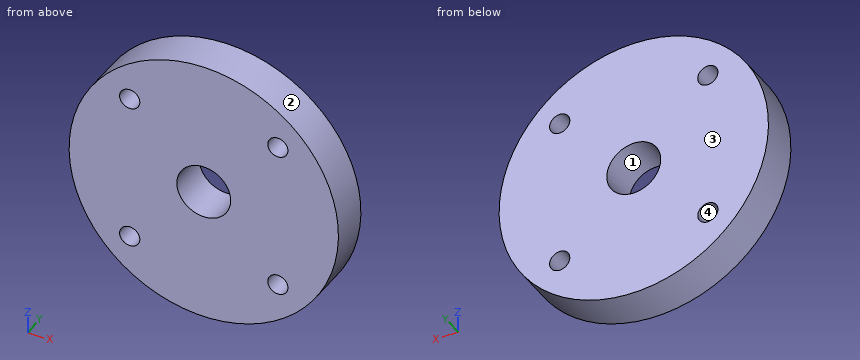
```python
from build123d import *

# Parameters (mm, degrees)
SKETCH1_R                         = 20
ARM_DISTANS_BOSS_EXTRUDE1_DEPTH   = 6
SKETCH2_R                         = 1.5
MOUNTING_HOLES_CUT_EXTRUDE1_DEPTH = 6
SKETCH3_R                         = 4
CUT_EXTRUDE1_DEPTH                = 6


with BuildPart() as part:
    # Sketch1 → Arm Distans Boss-Extrude1 (new body)
    with BuildSketch(Plane(origin=(0, 0, 0), x_dir=(1, 0, 0), z_dir=(0, 1, 0))):
        with Locations(Location((0, 0, 0), (0, 0, 270))):
            Circle(SKETCH1_R)
    extrude(amount=ARM_DISTANS_BOSS_EXTRUDE1_DEPTH)

    # Sketch2 → Mounting Holes Cut-Extrude1 (cut)
    with BuildSketch(Plane(origin=(0, 6, 0), x_dir=(1, 0, 0), z_dir=(0, 1, 0))):
        with Locations(Location((11, 11, 0), (0, 0, 270))):
            Circle(SKETCH2_R)
        with Locations(Location((-11, 11, 0), (0, 0, 270))):
            Circle(SKETCH2_R)
        with Locations(Location((-11, -11, 0), (0, 0, 270))):
            Circle(SKETCH2_R)
        with Locations(Location((11, -11, 0), (0, 0, 270))):
            Circle(SKETCH2_R)
    extrude(amount=-MOUNTING_HOLES_CUT_EXTRUDE1_DEPTH, mode=Mode.SUBTRACT)

    # Sketch3 → Cut-Extrude1 (cut)
    with BuildSketch(Plane.XZ):
        with Locations(Location((0, 0, 0), (0, 0, 270))):
            Circle(SKETCH3_R)
    extrude(amount=-CUT_EXTRUDE1_DEPTH, mode=Mode.SUBTRACT)


solid = part.part
```
Work out the finished part from the listing and answer in its coordinate system (mm). Face numbers are marked on the shaded views. Coordinates: 2 decimals unless noted, no trailing zeros. Loops run counter-clockwise (first coordinate to the right, second up) from the corner with the lowest first, then second, coordinate; pieces in that order, holes last. Notation, with made-up numbers: M -31,-15 L -19,-15 A15 cw -19,4 Z; hole C -1.5,59.5 d7. An arc over 180 degrees is marked long. Use CSV: the item, a comma, the result in double quotes. Start each with the question number.
(1) Consider line 1 (X direction, y = 1.8, z = -11); line 2 (X direction, y = 4.4, z = 0); line 3 (X direction, y = 3.75, z = -10.5). Determine where each line is inside the solid, lowest interval first.
(2) For a pull along Z with two mould halves and no side action, classify the marked faces 1, 2, 3 and 4 as +Z half, -Z half, draft (parallel to the pull), parting line (faces both ways), or undercut.
(3) Find section B-B, the plane z = -3. Give the vertices of the cut face in (x, y), then the cut area to 3 significant figures.
(4) Find section D-D, the plane x = 11. Give the vertices of the cut face in (y, z), then the cut area to 3 significant figures.
(5) Find section C-C, the plane y = 1.6. Give the vertices of the cut face in (x, z).
(6) Given pin 1 Ø3 at (x, y) = (2, 5.5) entering from -Z; pin 2 Ø1 at (x, y) = (12.5, 2) entering from +Z; pin 3 Ø1.5 at (y, z) = (1, 10.5) entering from -X, each flat-ended and moving along its own axis, determine where each tip first touches the part or whether it passes through.
(7) Find section A-A, the plane x = 0. Give the vertices of the cut face in (y, z), then the cut area to 3 significant figures.
Recorded:
1,line 1,"x = -16.7 to -12.5, -9.5 to 9.5, 12.5 to 16.7"
1,line 2,"x = -20 to -4, 4 to 20"
1,line 3,"x = -17.02 to -12.41, -9.59 to 9.59, 12.41 to 17.02"
2,face 1,"undercut"
2,face 2,"parting line"
2,face 3,"draft"
2,face 4,"undercut"
3,outline,"M -19.77,0 L -2.65,0 L -2.65,6 L -19.77,6 Z; M 2.65,0 L 19.77,0 L 19.77,6 L 2.65,6 Z"
3,area,"206 mm^2"
4,outline,"M 0,-16.7 L 6,-16.7 L 6,-12.5 L 0,-12.5 Z; M 0,-9.5 L 6,-9.5 L 6,9.5 L 0,9.5 Z; M 0,12.5 L 6,12.5 L 6,16.7 L 0,16.7 Z"
4,area,"164 mm^2"
5,outline,"C 0,0 d40; hole C -11,-11 d3; hole C -11,11 d3; hole C 0,0 d8; hole C 11,-11 d3; hole C 11,11 d3"
6,pin 1,"stops at z = -19.99"
6,pin 2,"stops at z = 16"
6,pin 3,"stops at x = -17.46"
7,outline,"M 0,-20 L 6,-20 L 6,-4 L 0,-4 Z; M 0,4 L 6,4 L 6,20 L 0,20 Z"
7,area,"192 mm^2"
